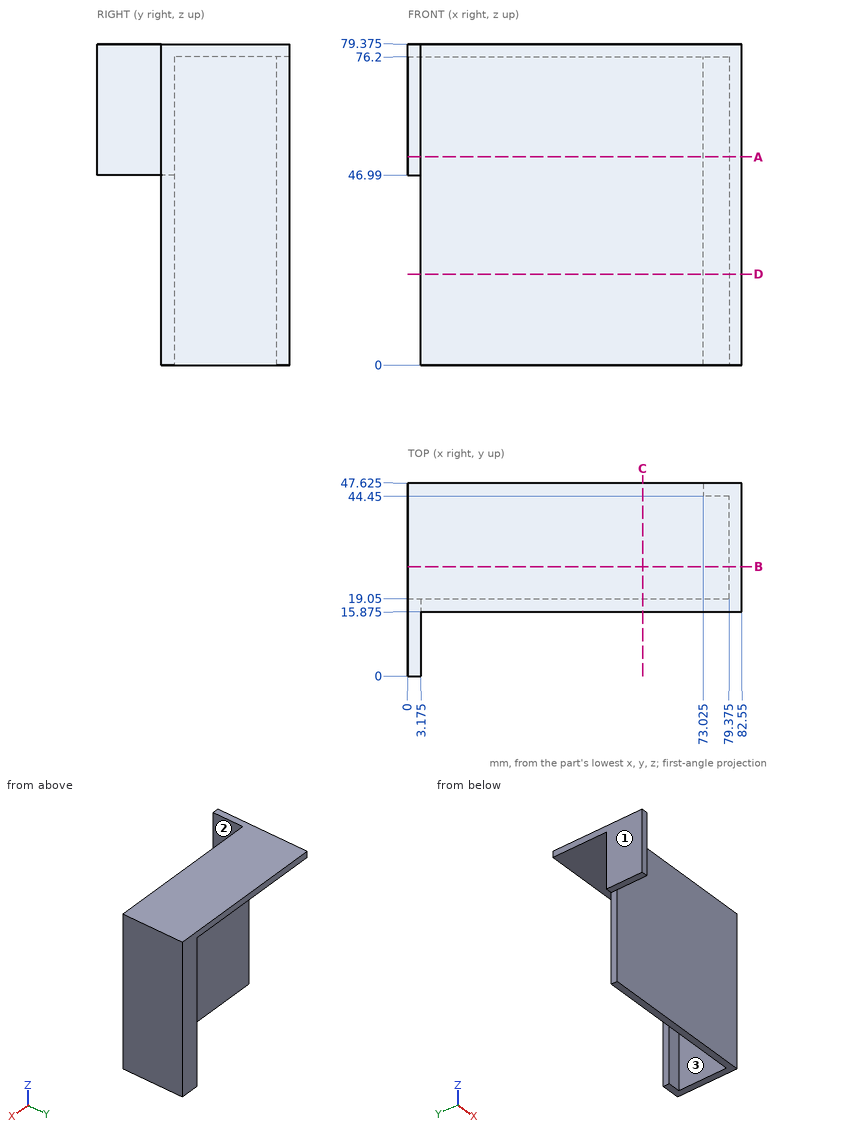
The drawing under review shows one solid part. Ordinate dimensions are in mm from its lowest x, y, z. A direction names the side the tool comes from. Round coordinates to 2 decimals unless told otherwise and drop trailing zeros. Order: outer loops, then holes, each group sorted by start corner. A loop starts at its lowest first (then second) coordinate and runs counter-clockwise, first axis right, second up. Notation, with made-up numbers: (-5.5, -16) -> (16.5, -16) arc R37 ccw to (16.5, 23) -> close; hole circle Ø9 at (-18, 62.25). An arc over 180 degrees is marked (long way). Use a Markdown table: item, result.
Q1. We need section C-C on x = 58. Write out the cut boundary in (y, z) (3 decimals), then the cut area to 3 significant figures.
Values:
| item | result |
|---|---|
| outline | (15.875, 0) -> (19.05, 0) -> (19.05, 76.2) -> (47.625, 76.2) -> (47.625, 79.375) -> (15.875, 79.375) -> close |
| area | 343 mm^2 |
Q2. We need section B-B on y = 27. Write out the cut boundary in (x, z) (3 decimals).
Values:
| item | result |
|---|---|
| outline | (0, 76.2) -> (79.375, 76.2) -> (79.375, 0) -> (82.55, 0) -> (82.55, 79.375) -> (0, 79.375) -> close |
Q3. We need section D-D on z = 22.5. Write out the cut boundary in (x, y) (3 decimals), then the cut area to 3 significant figures.
Values:
| item | result |
|---|---|
| outline | (3.175, 15.875) -> (82.55, 15.875) -> (82.55, 47.625) -> (73.025, 47.625) -> (73.025, 44.45) -> (79.375, 44.45) -> (79.375, 19.05) -> (3.175, 19.05) -> close |
| area | 363 mm^2 |
Q4. For line 1 (Y direction, x = 76, z = 31.5) (3 decimals); line 2 (X direction, y = 16, z = 10.5) (3 decimals); line 3 (Z direction, x = 8, y = 24) (3 decimals), list the stretches that pass through material, from the lowest coordinate up.
Values:
| item | result |
|---|---|
| line 1 | y = 15.875 to 19.05, 44.45 to 47.625 |
| line 2 | x = 3.175 to 82.55 |
| line 3 | z = 76.2 to 79.375 |
Q5. Tool access review of the marked faces 1, 2 and 3: name each direction out of +Z, -Z, +X, -X, +Y, -Y from which nothing blocks a thin tool from reaching the whole face with its end or side.
Values:
| item | result |
|---|---|
| face 1 | +Z, -Z, -X, +Y, -Y |
| face 2 | +Z, -Z, +X, -Y |
| face 3 | -Z, -X |
Q6. Clearance check with flat-ended pins moving along their axes: P1, Ø8, axis at y = 5, z = 59.5, coming from the +X side (3 decimals); P2, Ø1.6, axis at y = 17, z = 25.5, coming from the -X side (3 decimals); P3, Ø7, axis at x = 75.5, z = 29.5, coming from the -Y side (3 decimals). State where each tip first meets the part, or that it passes through.
Values:
| item | result |
|---|---|
| P1 | stops at x = 3.175 |
| P2 | stops at x = 3.175 |
| P3 | stops at y = 15.875 |
Q7. We need section A-A on z = 51.5. Write out the cut boundary in (x, y) (3 decimals), then the cut area to 3 significant figures.
Values:
| item | result |
|---|---|
| outline | (0, 0) -> (3.175, 0) -> (3.175, 15.875) -> (82.55, 15.875) -> (82.55, 47.625) -> (73.025, 47.625) -> (73.025, 44.45) -> (79.375, 44.45) -> (79.375, 19.05) -> (0, 19.05) -> close |
| area | 423 mm^2 |
